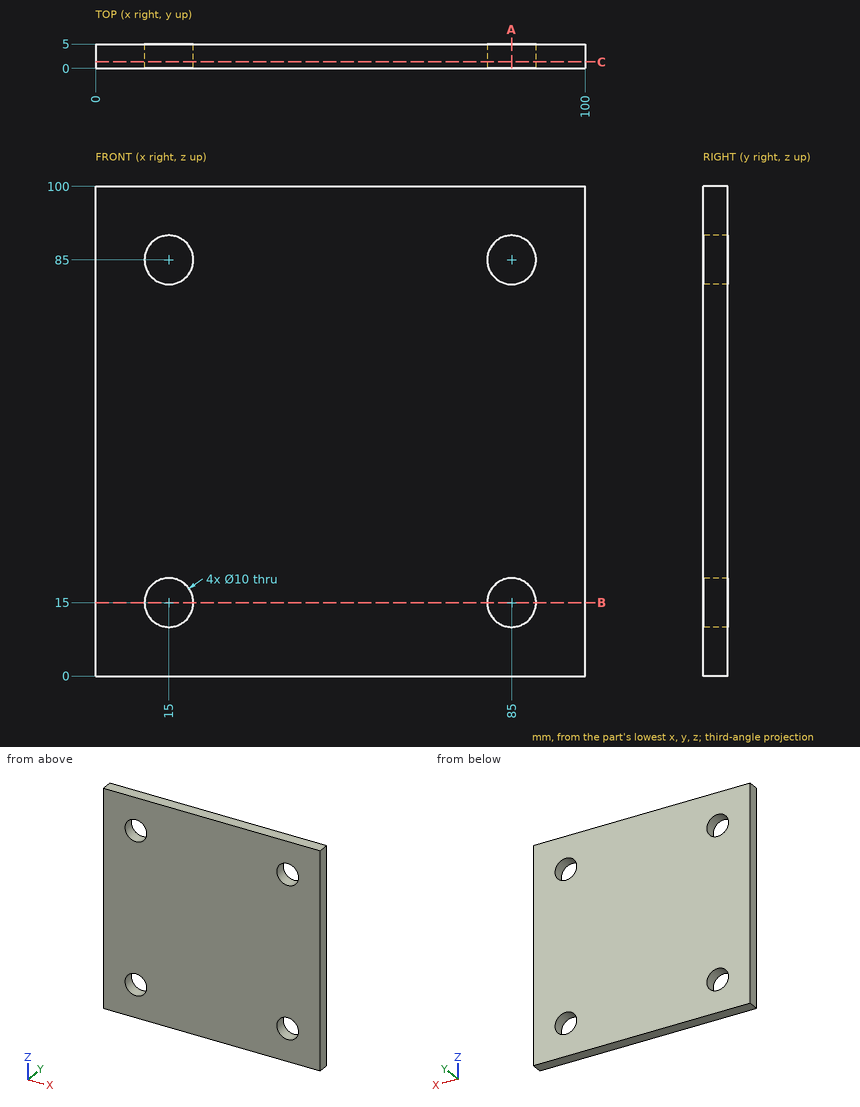
Design review of the part shown in the three views and the two pictorial views. Dimensions are in mm from the part's minimum x, y and z. Round coordinates to 2 decimals unless told otherwise and drop trailing zeros. Order: outer loops, then holes, each group sorted by start corner. A loop starts at its lowest first (then second) coordinate and runs counter-clockwise, first axis right, second up. Notation, with made-up numbers: (-19.75, 49) - (14.25, 49) arc R32 ccw to (14.25, 77) - close; hole circle Ø4 at (3.25, 38.5). An arc over 180 degrees is marked (long way). Answer in a Markdown table with one row per item.
(1) Take a section at C-C on y = 1.35. Write out the cut boundary in (x, z), plus the area to 3 significant figures.
Result set:
| item | result |
|---|---|
| outline | (0, 0) - (100, 0) - (100, 100) - (0, 100) - close; hole circle Ø10 at (15, 15); hole circle Ø10 at (15, 85); hole circle Ø10 at (85, 15); hole circle Ø10 at (85, 85) |
| area | 9,690 mm2 |
(2) Take a section at B-B on z = 15. Write out the cut boundary in (x, y).
Result set:
| item | result |
|---|---|
| outline | (0, 0) - (10, 0) - (10, 5) - (0, 5) - close; (20, 0) - (80, 0) - (80, 5) - (20, 5) - close; (90, 0) - (100, 0) - (100, 5) - (90, 5) - close |
(3) For line 1 (X direction, y = 2.65, z = 14.5); line 2 (Z direction, x = 15, y = 2.75); line 3 (Z direction, x = 12, y = 3.25), list the stretches that pass through material, from the lowest coordinate up. Write a range as from..to.
Result set:
| item | result |
|---|---|
| line 1 | x = 0..10.03, 19.97..80.03, 89.97..100 |
| line 2 | z = 0..10, 20..80, 90..100 |
| line 3 | z = 0..11, 19..81, 89..100 |
(4) Take a section at A-A on x = 85. Write out the cut boundary in (y, z), plus the area to 3 significant figures.
Result set:
| item | result |
|---|---|
| outline | (0, 0) - (5, 0) - (5, 10) - (0, 10) - close; (0, 20) - (5, 20) - (5, 80) - (0, 80) - close; (0, 90) - (5, 90) - (5, 100) - (0, 100) - close |
| area | 400 mm2 |
